Model file for the job. Use its own axes, mm. A direction names the side the tool comes from. Give positions to 0.01 mm unless a question says otherwise; leave off trailing zeros. Write each loop counter-clockwise with the first axis right and the second up, starting at its lowest first coordinate (ties: lowest second). Pieces come first, ordered by that corner, then holes. Notation, with made-up numbers: (16, 50.25) - (24, 50.25) arc R17 ccw to (24, 60.25) - close; hole circle Ø10 at (-34.75, -7). An arc over 180 degrees is marked (long way). One line per item, written item: value. Start each with the question number.
(1) Probe L1, parallel to Z at x = 21, y = -4.75; L2, parallel to Z at x = 45, y = -4.5; L3, parallel to X at y = -10, z = 94.5. List the from-to ranges inside material, lowest first.
(2) Cut at C-C, the plane y = -6.35. List the corners of the cut face in (x, z).
(3) 3-axis set-ups, long thin cutter, end or side, ignore diameter. For faces 4 (the face through (107.861, -5.689, 138.387)), 5 (the face through (63, -6, 127)), 6 (the face through (80.07, -8.32, 83.58)): which of +Z, -Z, +X, -X, +Y, -Y reach the whole face in a straight line?
(4) Drop flat-ended pins along their axis: P1, Ø11.5, axis at x = 32, z = 93.5, coming from the -Y side; P2, Ø2, axis at x = 41, y = -11, coming from the +Z side. Give the stop position or say it passes through.
(5) Cut at A-A, the plane z = 133.35. List the corners of the cut face in (x, y), and give its area (3 significant figures).
(6) Cut at D-D, the plane z = 107.5. List the corners of the cut face in (x, y).
(7) Mould opens along Z. For faces 1 (the face through (12.7, -6, 133)), 2 (the face through (101.6, -9.3, 129)), 3 (the face through (13, -6, 139.7)) say: pulls with the +Z half, pulls with the -Z half, needs draft (parallel to the pull), parting line crosses it, or undercut.
(8) Cut at B-B, the plane x = 60. List the corners of the cut face in (y, z).
from build123d import *

# Parameters (mm, degrees)
F0_W      = 127
F0_H      = 127
F1_DEPTH  = 12.7
F2_R      = 18.973851
F2_W      = 101.6
F2_H      = 50.8
F3_DEPTH  = 8.89
F4_W      = 25.4
F4_H      = 12.7
F5_DEPTH  = 12.7
F7_W      = 25.4
F7_H      = 12.7
F8_DEPTH  = 12.7
F9_R      = 5.08
F10_DEPTH = 12.7
F6_R      = 5.08
F11_DEPTH = 12.7


with BuildPart() as f1:
    # F0 (on Front) → F1 (new body)
    with BuildSketch(Plane.XZ):
        with Locations((63.5, 63.5)):
            Rectangle(F0_W, F0_H)
    extrude(amount=F1_DEPTH)

    # F2 (on face) → F3 (cut)
    with BuildSketch(Plane.XZ.offset(12.7)):
        with Locations((95.128258, 95.123877)):
            Circle(F2_R)
        with Locations((31.882087, 95.123877)):
            Circle(F2_R)
        with Locations((63.5, 31.75)):
            Rectangle(F2_W, F2_H)
    extrude(amount=-F3_DEPTH, mode=Mode.SUBTRACT)

    # F4 (on face) → F5 (join)
    with BuildSketch(Plane.XY.offset(127)):
        with Locations((12.7, -6.35)):
            Rectangle(F4_W, F4_H)
    extrude(amount=F5_DEPTH)

    # F7 (on face) → F8 (join)
    with BuildSketch(Plane.XY.offset(127)):
        with Locations((114.3, -6.35)):
            Rectangle(F7_W, F7_H)
    extrude(amount=F8_DEPTH)

    # F9 (on face) → F10 (cut)
    with BuildSketch(Plane(origin=(101.6, 0, 0), x_dir=(0, -1, 0), z_dir=(-1, 0, 0))):
        with Locations((6.35, 133.35)):
            Circle(F9_R)
    extrude(amount=-F10_DEPTH, mode=Mode.SUBTRACT)

    # F6 (on face) → F11 (cut)
    with BuildSketch(Plane.YZ.offset(25.4)):
        with Locations((-6.35, 133.35)):
            Circle(F6_R)
    extrude(amount=-F11_DEPTH, mode=Mode.SUBTRACT)


solid = f1.part
Answers follow:
1. L1: z = 0 to 6.35, 57.15 to 79.58, 110.67 to 128.53, 138.17 to 139.7
1. L2: z = 0 to 6.35, 57.15 to 81.42, 108.83 to 127
1. L3: x = 0 to 12.92, 50.85 to 76.16, 114.09 to 127
2. outline: (0, 0) - (127, 0) - (127, 139.7) - (101.6, 139.7) - (101.6, 138.43) - (114.3, 138.43) - (114.3, 128.27) - (101.6, 128.27) - (101.6, 127) - (25.4, 127) - (25.4, 128.27) - (12.7, 128.27) - (12.7, 138.43) - (25.4, 138.43) - (25.4, 139.7) - (0, 139.7) - close; hole (12.7, 6.35) - (114.3, 6.35) - (114.3, 57.15) - (12.7, 57.15) - close; hole circle Ø37.95 at (31.88, 95.12); hole circle Ø37.95 at (95.13, 95.12)
3. face 4: none
3. face 5: +Z, +Y, -Y
3. face 6: -Y
4. P1: stops at y = -3.81
4. P2: stops at z = 127
5. outline: (0, -12.7) - (25.4, -12.7) - (25.4, -11.43) - (12.7, -11.43) - (12.7, -1.27) - (25.4, -1.27) - (25.4, 0) - (0, 0) - close; (101.6, -12.7) - (127, -12.7) - (127, 0) - (101.6, 0) - (101.6, -1.27) - (114.3, -1.27) - (114.3, -11.43) - (101.6, -11.43) - close
5. area: 387 mm²
6. outline: (0, -12.7) - (17.5, -12.7) - (17.5, -3.81) - (46.26, -3.81) - (46.26, -12.7) - (80.75, -12.7) - (80.75, -3.81) - (109.51, -3.81) - (109.51, -12.7) - (127, -12.7) - (127, 0) - (0, 0) - close
7. face 1: undercut
7. face 2: needs draft
7. face 3: pulls with the +Z half
8. outline: (-12.7, 0) - (0, 0) - (0, 127) - (-12.7, 127) - (-12.7, 57.15) - (-3.81, 57.15) - (-3.81, 6.35) - (-12.7, 6.35) - close
